Source: CAD feature listing. Evaluate the final solid. Frame: model axes, mm. A direction names the side the tool comes from. Coordinates: 2 decimals unless noted, no trailing zeros. Order: outer loops, then holes, each group sorted by start corner. A loop starts at its lowest first (then second) coordinate and runs counter-clockwise, first axis right, second up. Notation, with made-up numbers: (6, 29) - (34, 29) arc R21 ccw to (34, 49) - close; hole circle Ø10 at (17.5, -33). An arc over 180 degrees is marked (long way). One line per question, with ' | ' between items. Start each with the question number.
(1) Access query for faces 3 (the flat face through (26, 8, 23.5)), 4 (the flat face through (10, 10, -5.5)), 5 (the cylindrical face through (17.21, 33.226, 11.661)). Directions: +Z, -Z, +X, -X, +Y, -Y. A direction counts if a zero-diameter tool reaches every point of the face in a straight line with its end or side. Return the directions, or none.
(2) Contact query for flat-ended pins moving along their axis: P1, Ø4, axis at x = -37, y = 0, coming from the +Z side; P2, Ø3, axis at y = -1.5, z = 7, coming from the +X side; P3, Ø3, axis at y = 10, z = -5, coming from the +X side; P4, Ø8, axis at x = 12.5, z = 8.5, coming from the -Y side. Output: stop coordinate, or through.
(3) Draft query along Y for faces 1 (the flat face through (8, 26, 23.5)), 2 (the flat face through (0, -24, 35.5)). Return one class per face: +Y half, -Y half, draft (parallel to the pull), parting line (faces both ways), or undercut.
(4) Section A-A (z = 6.5). Count the separate pieces of the cut face and the enclosed holes in it, then the cut area to 3 significant figures.
(5) Section D-D (z = -10). Return the cut outline in (x, y), then the cut area to 3 significant figures.
(6) Section C-C (x = -37). Return the cut outline in (y, z), then the cut area to 3 significant figures.
(7) Line query: line 1 along Y through (x, z) = (-0.5, 6); line 2 along Y through (x, z) = (-22, 32.5); line 3 along X through (y, z) = (-30.5, 11.5). Output: solid intervals per line, ascending.
from build123d import *

# Parameters (mm, degrees)
SKETCH_1_R               = 42
EXTRUDE_1_DEPTH          = 10
SKETCH_2_R               = 40
EXTRUDE_2_DEPTH          = 13
SKETCH_3_R               = 32
EXTRUDE_3_DEPTH          = 12.5
SKETCH_4_R               = 22.5
EXTRUDE_4_DEPTH          = 8.5
EXTRUDE_START            = 5.5
SKETCH_5_R               = 22.5
EXTRUDE_5_DEPTH          = 5.5
SKETCH_6_R               = 12.5
EXTRUDE_6_DEPTH          = 7
SKETCH_7_R               = 9.5
CUT_EXTRUDE_1_DEPTH      = 56.5
SKETCH_8_R               = 1.75
CUT_EXTRUDE_2_DEPTH      = 23
SKETCH_9_R               = 1.75
CUT_EXTRUDE_3_DEPTH      = 12
CUT_EXTRUDE_4_REACH      = 83.672
CUT_EXTRUDE_4_END_RADIUS = 9.5
SKETCH_11_R              = 1.5
PATTERN_CIRCULAR_1_COUNT = 3


with BuildPart() as part:
    # Эскиз1 → Бобышка-Вытянуть1 (new body)
    with BuildSketch(Plane.XY):
        Circle(SKETCH_1_R)
    extrude(amount=EXTRUDE_1_DEPTH)

    # Эскиз2 → Бобышка-Вытянуть2 (add)
    with BuildSketch(Plane.XY.offset(10)):
        with Locations(Location((0, 0, 0), (0, 0, 180))):
            Circle(SKETCH_2_R)
    extrude(amount=EXTRUDE_2_DEPTH)

    # Эскиз3 → Бобышка-Вытянуть3 (add)
    with BuildSketch(Plane.XY.offset(23)):
        Circle(SKETCH_3_R)
    extrude(amount=EXTRUDE_3_DEPTH)

    # Эскиз4 → Бобышка-Вытянуть4 (add)
    with BuildSketch(Plane.XY.offset(35.5)):
        Circle(SKETCH_4_R)
    extrude(amount=EXTRUDE_4_DEPTH)

    # Эскиз5 → Бобышка-Вытянуть5 (add)
    with BuildSketch(Plane(origin=(0, 0, 0), x_dir=(-1, 0, 0), z_dir=(0, 0, -1)).offset(EXTRUDE_START)):
        with Locations(Location((0, 0, 0), (0, 0, 180))):
            Circle(SKETCH_5_R)
    extrude(amount=-EXTRUDE_5_DEPTH)

    # Эскиз6 → Бобышка-Вытянуть6 (add)
    with BuildSketch(Plane(origin=(0, 0, -5.5), x_dir=(-1, 0, 0), z_dir=(0, 0, -1))):
        Circle(SKETCH_6_R)
    extrude(amount=EXTRUDE_6_DEPTH)

    # Эскиз7 → Вырез-Вытянуть1 (cut)
    with BuildSketch(Plane(origin=(0, 0, -12.5), x_dir=(-1, 0, 0), z_dir=(0, 0, -1))):
        Circle(SKETCH_7_R)
    extrude(amount=-CUT_EXTRUDE_1_DEPTH, mode=Mode.SUBTRACT)

    # Эскиз8 → Вырез-Вытянуть2 (cut)
    with BuildSketch(Plane.XY.offset(23)):
        with Locations((0, 37)):
            Circle(SKETCH_8_R)
        with Locations((18.5, 32.04293994)):
            Circle(SKETCH_8_R)
        with Locations((32.04293994, 18.5)):
            Circle(SKETCH_8_R)
        with Locations((37, 0)):
            Circle(SKETCH_8_R)
        with Locations((32.04293994, -18.5)):
            Circle(SKETCH_8_R)
        with Locations((18.5, -32.04293994)):
            Circle(SKETCH_8_R)
        with Locations((0, -37)):
            Circle(SKETCH_8_R)
        with Locations((-18.5, -32.04293994)):
            Circle(SKETCH_8_R)
        with Locations((-32.04293994, -18.5)):
            Circle(SKETCH_8_R)
        with Locations((-37, 0)):
            Circle(SKETCH_8_R)
        with Locations((-32.04293994, 18.5)):
            Circle(SKETCH_8_R)
        with Locations((-18.5, 32.04293994)):
            Circle(SKETCH_8_R)
    extrude(amount=-CUT_EXTRUDE_2_DEPTH, mode=Mode.SUBTRACT)

    # Эскиз9 → Вырез-Вытянуть3 (cut)
    with BuildSketch(Plane.XY.offset(35.5)):
        with Locations((-8.343458848, 25.67852594)):
            Circle(SKETCH_9_R)
        with Locations((8.343458848, 25.67852594)):
            Circle(SKETCH_9_R)
        with Locations((15.870201812, 21.843458848)):
            Circle(SKETCH_9_R)
        with Locations((21.843458848, 15.870201812)):
            Circle(SKETCH_9_R)
        with Locations((25.67852594, 8.343458848)):
            Circle(SKETCH_9_R)
        with Locations((25.67852594, -8.343458848)):
            Circle(SKETCH_9_R)
        with Locations((21.843458848, -15.870201812)):
            Circle(SKETCH_9_R)
        with Locations((15.870201812, -21.843458848)):
            Circle(SKETCH_9_R)
        with Locations((8.343458848, -25.67852594)):
            Circle(SKETCH_9_R)
        with Locations((-8.343458848, -25.67852594)):
            Circle(SKETCH_9_R)
        with Locations((-15.870201812, -21.843458848)):
            Circle(SKETCH_9_R)
        with Locations((-21.843458848, -15.870201812)):
            Circle(SKETCH_9_R)
        with Locations((-25.67852594, -8.343458848)):
            Circle(SKETCH_9_R)
        with Locations((-25.67852594, 8.343458848)):
            Circle(SKETCH_9_R)
        with Locations((-21.843458848, 15.870201812)):
            Circle(SKETCH_9_R)
        with Locations((-15.870201812, 21.843458848)):
            Circle(SKETCH_9_R)
    extrude(amount=-CUT_EXTRUDE_3_DEPTH, mode=Mode.SUBTRACT)

    # Вырез-Вытянуть4: up to this cylinder (the profile starts outside it)
    cut_extrude_4_end = Plane(origin=(0, 0, -10), z_dir=(0, 0, -1)) * Cylinder(CUT_EXTRUDE_4_END_RADIUS, 187.344, mode=Mode.PRIVATE)
    # Эскиз11 → Вырез-Вытянуть4 (cut, up to the surface)
    with BuildSketch(Plane(origin=(0, 12.5, 0), x_dir=(1, 0, 0), z_dir=(0, 1, 0)), mode=Mode.PRIVATE) as cut_extrude_4_sk1:
        with Locations(Location((0, 10, 0), (0, 0, 270))):
            Circle(SKETCH_11_R)
    cut_extrude_4_tool1 = extrude(cut_extrude_4_sk1.sketch, amount=-CUT_EXTRUDE_4_REACH, mode=Mode.PRIVATE) - cut_extrude_4_end
    cut_extrude_4 = cut_extrude_4_tool1.solids().sort_by_distance((0, 12.5, -10))[0]
    add(cut_extrude_4, mode=Mode.SUBTRACT)

    # Круговой массив1: Вырез-Вытянуть4 ×3 about axis
    pattern_circular_1_axis = Axis((0, 0, 70.870057685), (0, 0, -1))
    for i in range(1, PATTERN_CIRCULAR_1_COUNT):
        add(cut_extrude_4.rotate(pattern_circular_1_axis, i * 360 / PATTERN_CIRCULAR_1_COUNT), mode=Mode.SUBTRACT)


solid = part.part
Response values:
1) face 3: +Z | face 4: -Z | face 5: +Z, -Z
2) P1: stops at z = 23 | P2: stops at x = 42 | P3: stops at x = 20.83 | P4: stops at y = -41.13
3) face 1: undercut | face 2: draft
4) separate pieces: 1 | enclosed holes: 13 | area: 5,140 mm²
5) outline: (-11.5, -4.91) - (-8.87, -3.39) arc R9.5 cw to (-1.5, 9.38) - (-1.5, 12.41) arc R12.5 ccw to start; (-10, -7.5) arc R12.5 ccw to (10, -7.5) - (7.37, -5.99) arc R9.5 cw to (-7.37, -5.99) - close; (1.5, 9.38) arc R9.5 cw to (8.87, -3.39) - (11.5, -4.91) arc R12.5 ccw to (1.5, 12.41) - close | area: 180 mm²
6) outline: (-19.87, 0) - (-1.75, 0) - (-1.75, 23) - (-15.2, 23) - (-15.2, 10) - (-19.87, 10) - close; (1.75, 0) - (19.87, 0) - (19.87, 10) - (15.2, 10) - (15.2, 23) - (1.75, 23) - close | area: 712 mm²
7) line 1: y = -42 to -38.68, -35.32 to -9.49, 9.49 to 35.32, 38.68 to 42 | line 2: y = -23.24 to -17.61, -14.13 to 14.13, 17.61 to 23.24 | line 3: x = -25.88 to -19.33, -17.67 to 17.67, 19.33 to 25.88
